from build123d import *

# Parameters (mm, degrees)
BOSS_EXTRUDE1_DEPTH = 400
FILLET1_R           = 20
CUT_EXTRUDE1_START  = -20
CUT_EXTRUDE1_DEPTH  = 360


with BuildPart() as part:
    # Sketch1 → Boss-Extrude1 (new body)
    with BuildSketch(Plane(origin=(0, 0, 0), x_dir=(1, 0, 0), z_dir=(0, 1, 0))):
        with BuildLine():
            Line((0, 960), (0, 1460))
            ThreePointArc((0, 1460), (558.717811253, 1348.864117466), (1032.375900532, 1032.375900532))
            Line((1032.375900532, 1032.375900532), (678.822509939, 678.822509939))
            ThreePointArc((678.822509939, 678.822509939), (367.37609507, 886.924351211), (0, 960))
        make_face()
    extrude(amount=BOSS_EXTRUDE1_DEPTH)

    # Fillet1
    fillet1_edges = [part.edges().sort_by_distance(p)[0] for p in [
        (367.37609507, 400, -886.924351211),
        (855.599205236, 400, -855.599205236),
        (558.717811253, 400, -1348.864117466),
        (1032.375900532, 200, -1032.375900532),
        (678.822509939, 200, -678.822509939),
        (0, 200, -960),
        (0, 200, -1460),
        (0, 400, -1210),
    ]]
    fillet(fillet1_edges, radius=FILLET1_R)

    # Sketch4 → Cut-Extrude1 (cut)
    with BuildSketch(Plane(origin=(0, 400, 0), x_dir=(1, 0, 0), z_dir=(0, 1, 0)).offset(CUT_EXTRUDE1_START)):
        with BuildLine():
            ThreePointArc((20, 979.795897113), (375.029763718, 905.401941861), (678.678187404, 706.962458651))
            Line((678.678187404, 706.962458651), (1003.993415273, 1032.277686521))
            ThreePointArc((1003.993415273, 1032.277686521), (551.064142606, 1330.386526816), (20, 1439.861104413))
            Line((20, 1439.861104413), (20, 979.795897113))
        make_face()
    extrude(amount=-CUT_EXTRUDE1_DEPTH, mode=Mode.SUBTRACT)


solid = part.part
Here's how the part is built. I have some questions about the finished solid (model axes, mm). A direction names the side the tool comes from. Round coordinates to 2 decimals unless told otherwise and drop trailing zeros. Order: outer loops, then holes, each group sorted by start corner. A loop starts at its lowest first (then second) coordinate and runs counter-clockwise, first axis right, second up. Notation, with made-up numbers: (-0.75, -36.5) -> (45.25, -36.5) arc R25 ccw to (45.25, -22.5) -> close; hole circle Ø1 at (80, 22.25). An arc over 180 degrees is marked (long way). Return JSON: item names as keys, results as strings.
Q1. If we section it at A-A on y = 278: List the corners of the cut face in (x, z) for me.
Filled sheet:
{"outline": "(0, -1439.86) arc R20 ccw to (20.28, -1459.86) arc R1460 ccw to (1017.94, -1046.61) arc R20 ccw to (1018.14, -1018.14) -> (692.82, -692.82) arc R20 ccw to (664.83, -692.53) arc R960 cw to (19.59, -959.8) arc R20 ccw to (0, -979.8) -> close; hole (20, -1439.86) arc R1440 ccw to (1003.99, -1032.28) -> (678.68, -706.96) arc R980 cw to (20, -979.8) -> close"}
Q2. Which directions (+Z, -Z, +X, -X, +Y, -Y) give clear straight access to the entire face, cutting with the end or side of a thin tool? Please do faces 1 (the flat face through (505, 20, -1079)), 2 (the cylindrical face through (1023.99, 192.66, -1032.64)).
Filled sheet:
{"face 1": "none", "face 2": "+X, +Y, -Y"}
Q3. If we mould it in two halves opening along Y, with no side actions, what happens to faces 3 (the cylindrical face through (849.168, 393.986, -857.234)), 4 (the cylindrical face through (371.99, 187.34, -885)), 5 (the flat face through (519, 0, -1079)), 6 (the flat face through (839.059, 202.52, -867.343))? For each: released by +Y, released by -Y, zero draft, split by the parting line, or undercut.
Filled sheet:
{"face 3": "released by +Y", "face 4": "zero draft", "face 5": "released by -Y", "face 6": "undercut"}
Q4. For pin 1 Ø6 at (y, z) = (313.5, -845) entering from +X; pin 2 Ø1.5 at (y, z) = (83, -1181) entering from +X; pin 3 Ø5 at (x, y) = (774.5, 279) entering from +Z; pin 4 Ø8 at (x, z) = (521, -1166.5) entering from -Y, each with a flat end and sliding along its axis, tell me the tip position at first contact or that it passes through.
Filled sheet:
{"pin 1": "stops at x = 848", "pin 2": "stops at x = 859.42", "pin 3": "stops at z = -772", "pin 4": "stops at y = 0"}
Q5. I need wall thicknesses on line 1 along Y through (x, z) = (455, -1290); line 2 along Z through (x, y) = (301, 177); line 3 along X through (y, z) = (86, -1238). Which ranges of each line are inside material? Lowest first, please. Write a range as from..to.
Filled sheet:
{"line 1": "y = 0..20, 380..400", "line 2": "z = -1428.64..-1408.19, -932.63..-911.59", "line 3": "x = 0..20, 735.5..773.92"}
